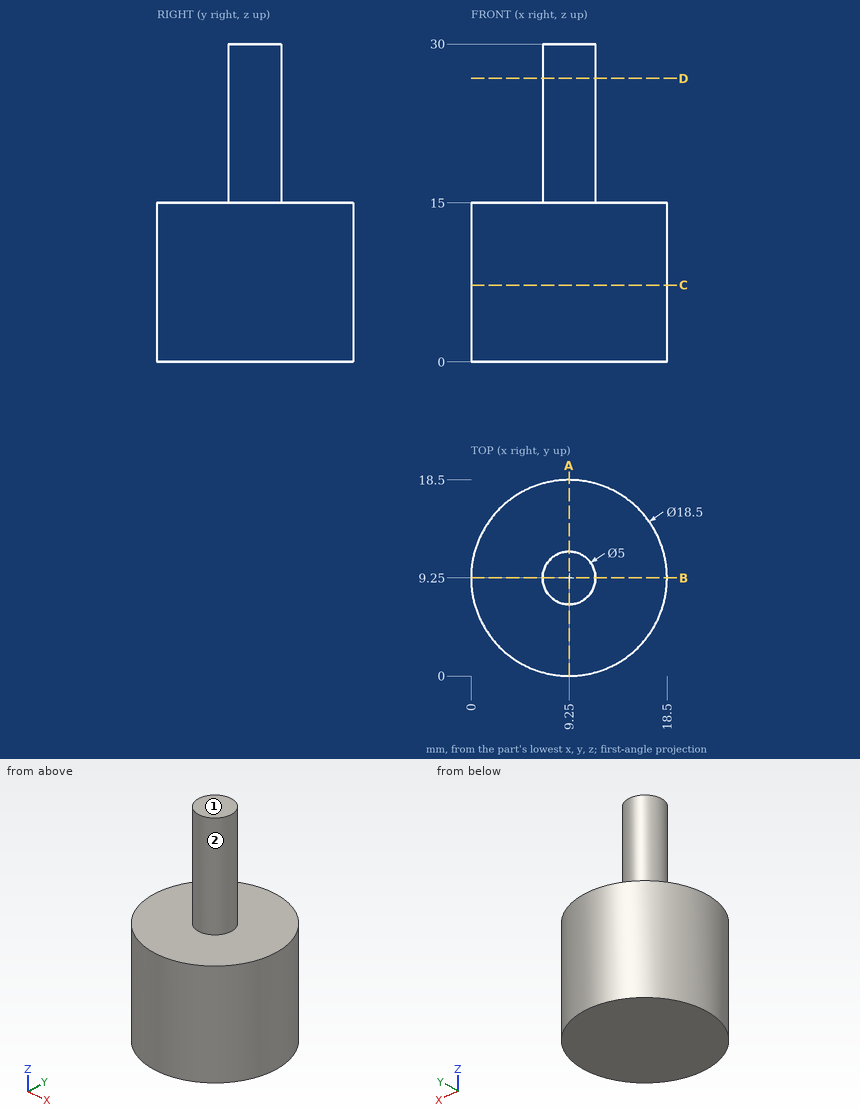
Geometry: see drawing. Coordinates: mm, zero at the bounding-box minimum. A direction names the side the tool comes from. Give positions to 0.01 mm unless a question says otherwise; leave off trailing zeros. Loops run counter-clockwise (first coordinate to the right, second up) from the corner with the lowest first, then second, coordinate; pieces in that order, holes last. Notation, with made-up numbers: (62, -4.75) -> (94, -4.75) arc R20 cw to (94, 15.25) -> close; hole circle Ø7 at (40, 87). An arc over 180 degrees is marked (long way). Answer as a JSON object with one key per item and string values. Group by question number.
Item 1: Cut plane A-A, the plane x = 9.25. Return the cut outline in (y, z), and give its area (4 significant figures).
Item 2: Cut plane C-C, the plane z = 7.25. Return the cut outline in (x, y).
Item 3: Line query: probe 1 along Z at (x, y) = (15, 9.25); probe 2 along X at (y, z) = (10.75, 26); probe 3 along Y at (x, z) = (17.5, 1.5). Output: solid intervals per line, ascending.
Item 4: Pin query (flat end, axial travel): P1, Ø10, axis at x = 9.5, z = 21, coming from the +Y side; P2, Ø6, axis at x = 4, z = 17.5, coming from the +Y side; P3, Ø1.5, axis at x = 13, z = 10.5, coming from the -Y side. Return the tip coordinate at first contact, or that it passes through.
Item 5: Cut plane D-D, the plane z = 26.75. Return the cut outline in (x, y), and give its area (3 significant figures).
Item 6: Reachability of the marked faces 1 and 2 from +Z, -Z, +X, -X, +Y, -Y: full face, straight path, thin tool, end or side. Return the list, or none.
Checks:
{
 "1": {"outline": "(0, 0) -> (18.5, 0) -> (18.5, 15) -> (11.75, 15) -> (11.75, 30) -> (6.75, 30) -> (6.75, 15) -> (0, 15) -> close", "area": "352.5 mm²"},
 "2": {"outline": "circle Ø18.5 at (9.25, 9.25)"},
 "3": {"probe 1": "z = 0 to 15", "probe 2": "x = 7.25 to 11.25", "probe 3": "y = 5.07 to 13.43"},
 "4": {"P1": "stops at y = 11.75", "P2": "stops at y = 17.77", "P3": "stops at y = 0.5"},
 "5": {"outline": "circle Ø5 at (9.25, 9.25)", "area": "19.6 mm²"},
 "6": {"face 1": "+Z, +X, -X, +Y, -Y", "face 2": "+Z"}
}
